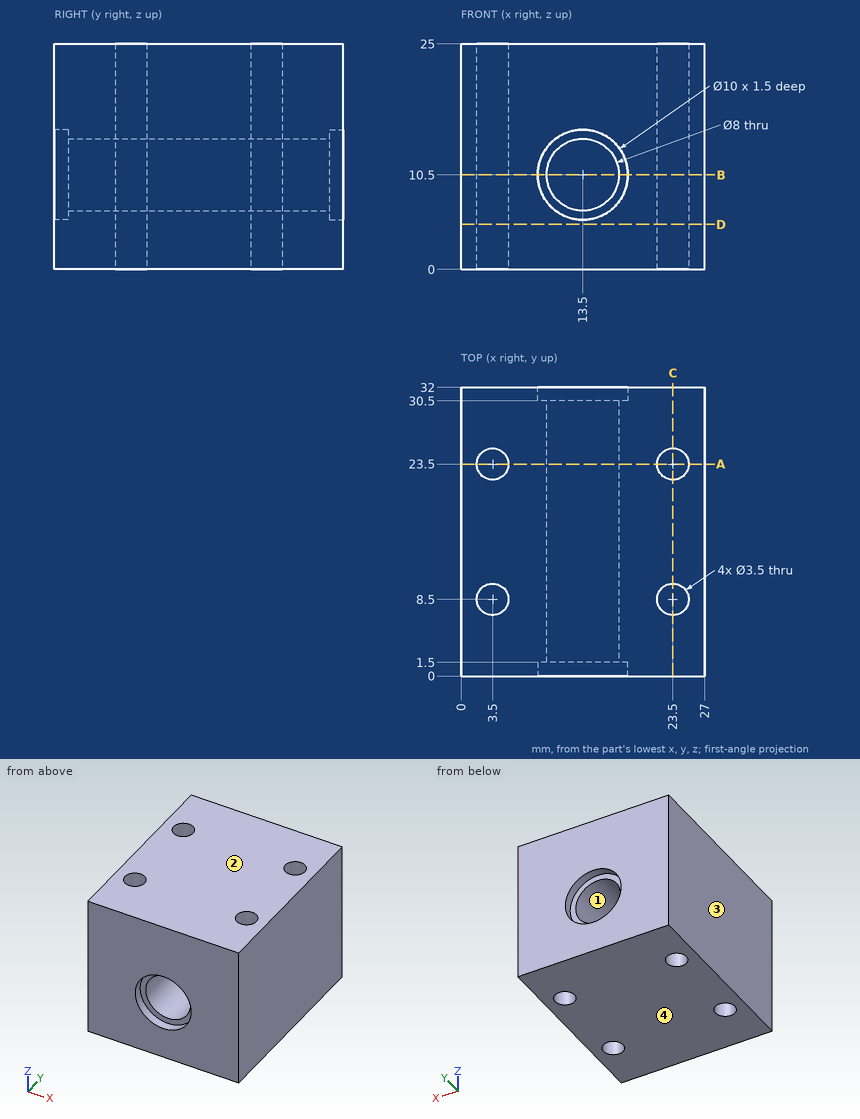
Print and shaded views of the part. All mm, measured from the part's lowest x, y and z. Give positions to 0.01 mm unless a question says otherwise; leave off trailing zeros. Loops run counter-clockwise (first coordinate to the right, second up) from the corner with the lowest first, then second, coordinate; pieces in that order, holes last.
1) Pull direction Z, two halves, no side cores. Call the marked faces 1, 2, 3 and 4: +Z half, -Z half, draft (parallel to the pull), parting line (faces both ways), or undercut.
2) Saw through at C-C (x = 23.5). Write the cut outline in (y, z), plus the area to 3 significant figures.
3) Saw through at A-A (y = 23.5). Write the cut outline in (x, z), plus the area to 3 significant figures.
4) Wall check: line 1 (Y direction, x = 23.5, z = 12.25); line 2 (X direction, y = 10.75, z = 10.5); line 3 (Y direction, x = 24.25, z = 14.25). Give the ranges that are in metal, low to high.
5) Saw through at B-B (z = 10.5). Write the cut outline in (x, y), plus the area to 3 significant figures.
6) Flat gauge pins, fed straight in: pin 1 Ø9 at (x, z) = (13.5, 10.5) entering from -Y; pin 2 Ø2 at (x, y) = (3.5, 8.5) entering from -Z. Where does each tip first touch, or does it go through?
7) Saw through at D-D (z = 5). Write the cut outline in (x, y), plus the area to 3 significant figures.
Answer block:
1. face 1: undercut
1. face 2: +Z half
1. face 3: draft
1. face 4: -Z half
2. outline: (0, 0) - (6.75, 0) - (6.75, 25) - (0, 25) - close; (10.25, 0) - (21.75, 0) - (21.75, 25) - (10.25, 25) - close; (25.25, 0) - (32, 0) - (32, 25) - (25.25, 25) - close
2. area: 625 mm2
3. outline: (0, 0) - (1.75, 0) - (1.75, 25) - (0, 25) - close; (5.25, 0) - (21.75, 0) - (21.75, 25) - (5.25, 25) - close; (25.25, 0) - (27, 0) - (27, 25) - (25.25, 25) - close; hole circle Ø8 at (13.5, 10.5)
3. area: 450 mm2
4. line 1: y = 0 to 6.75, 10.25 to 21.75, 25.25 to 32
4. line 2: x = 0 to 9.5, 17.5 to 27
4. line 3: y = 0 to 6.92, 10.08 to 21.92, 25.08 to 32
5. outline: (0, 0) - (8.5, 0) - (8.5, 1.5) - (9.5, 1.5) - (9.5, 30.5) - (8.5, 30.5) - (8.5, 32) - (0, 32) - close; (17.5, 1.5) - (18.5, 1.5) - (18.5, 0) - (27, 0) - (27, 32) - (18.5, 32) - (18.5, 30.5) - (17.5, 30.5) - close; hole circle Ø3.5 at (3.5, 8.5); hole circle Ø3.5 at (3.5, 23.5); hole circle Ø3.5 at (23.5, 8.5); hole circle Ø3.5 at (23.5, 23.5)
5. area: 564 mm2
6. pin 1: stops at y = 1.5
6. pin 2: passes through
7. outline: (0, 0) - (27, 0) - (27, 32) - (0, 32) - close; hole circle Ø3.5 at (3.5, 8.5); hole circle Ø3.5 at (3.5, 23.5); hole circle Ø3.5 at (23.5, 8.5); hole circle Ø3.5 at (23.5, 23.5)
7. area: 826 mm2
